from build123d import *

# Parameters (mm, degrees)
SKETCH1_R                 = 1.27
SKETCH1_R_2               = 1.5875
BOSS_EXTRUDE1_DEPTH       = 1.5875
CUT_EXTRUDE3_DEPTH        = 163.771012948
CUT_EXTRUDE4_DEPTH        = 163.771012948
F_8_0MM_DOWEL_HOLE1_D     = 8
F_8_0MM_DOWEL_HOLE1_DEPTH = 5.08
F_8_0MM_DOWEL_HOLE1_TIP   = 2.403442476


with BuildPart() as part:
    # Sketch1 → Boss-Extrude1 (new body)
    with BuildSketch(Plane(origin=(0, 0, 0), x_dir=(1, 0, 0), z_dir=(0, 1, 0))):
        with BuildLine():
            Line((-152.4, 43.5), (-152.4, -7.3))
            ThreePointArc((-152.4, -7.3), (-148.680256121, -16.280256121), (-139.7, -20))
            Line((-139.7, -20), (-61.723030548, -20))
            ThreePointArc((-61.723030548, -20), (-55.173880707, -21.818886254), (-50.500661357, -26.754545455))
            ThreePointArc((-50.500661357, -26.754545455), (57.15, 0), (-50.500661357, 26.754545455))
            ThreePointArc((-50.500661357, 26.754545455), (-55.173880707, 21.818886254), (-61.723030548, 20))
            Line((-61.723030548, 20), (-88.9, 20))
            ThreePointArc((-88.9, 20), (-97.880256121, 23.719743879), (-101.6, 32.7))
            Line((-101.6, 32.7), (-101.6, 43.5))
            ThreePointArc((-101.6, 43.5), (-105.319743879, 52.480256121), (-114.3, 56.2))
            Line((-114.3, 56.2), (-139.7, 56.2))
            ThreePointArc((-139.7, 56.2), (-148.680256121, 52.480256121), (-152.4, 43.5))
        make_face()
        with Locations(Location((-136.8, 0, 0), (0, 0, 270))):
            Circle(SKETCH1_R, mode=Mode.SUBTRACT)
        with Locations(Location((-117.2, 0, 0), (0, 0, 270))):
            Circle(SKETCH1_R, mode=Mode.SUBTRACT)
        with Locations(Location((0, 0, 0), (0, 0, 270))):
            Circle(SKETCH1_R_2, mode=Mode.SUBTRACT)
        with BuildLine():
            Line((-139.7, 33.02), (-114.3, 33.02))
            ThreePointArc((-114.3, 33.02), (-109.22, 38.1), (-114.3, 43.18))
            Line((-114.3, 43.18), (-139.7, 43.18))
            ThreePointArc((-139.7, 43.18), (-144.78, 38.1), (-139.7, 33.02))
        make_face(mode=Mode.SUBTRACT)
    extrude(amount=BOSS_EXTRUDE1_DEPTH)

    # Sketch5 → Cut-Extrude3 (cut, through all)
    with BuildSketch(Plane.XZ):
        with BuildLine():
            ThreePointArc((-19.811942673, -0.047660352), (-9.947246413, 17.133815477), (9.864696261, 17.18147583))
            ThreePointArc((9.864696261, 17.18147583), (14.025645813, 18.307134225), (12.899987418, 22.468083777))
            ThreePointArc((12.899987418, 22.468083777), (-13.007937617, 22.405758701), (-25.907925034, -0.062325076))
            ThreePointArc((-25.907925034, -0.062325076), (-22.852601492, -3.102983895), (-19.811942673, -0.047660352))
        make_face()
    extrude(amount=-CUT_EXTRUDE3_DEPTH, mode=Mode.SUBTRACT)

    # Sketch6 → Cut-Extrude4 (cut, through all)
    with BuildSketch(Plane.XZ):
        with BuildLine():
            Line((-16.102923339, -12.651081374), (-25.638527302, -29.167231918))
            ThreePointArc((-25.638527302, -29.167231918), (-26.310404552, -33.838744139), (-23.573299486, -37.683572006))
            Line((-23.573299486, -37.683572006), (-20.6375, -35.745198541))
            Line((-20.6375, -35.745198541), (-20.848318298, -39.257484944))
            ThreePointArc((-20.848318298, -39.257484944), (-17.010278569, -41.06644522), (-13.017246571, -42.501221061))
            Line((-13.017246571, -42.501221061), (-10.682756087, -39.86858848))
            Line((-10.682756087, -39.86858848), (-9.977344313, -43.315760417))
            ThreePointArc((-9.977344313, -43.315760417), (-5.801889244, -44.069724088), (-1.5735692, -44.422138399))
            Line((-1.5735692, -44.422138399), (0, -41.275))
            Line((0, -41.275), (1.5735692, -44.422138399))
            ThreePointArc((1.5735692, -44.422138399), (5.801889244, -44.069724088), (9.977344313, -43.315760417))
            Line((9.977344313, -43.315760417), (10.682756087, -39.86858848))
            Line((10.682756087, -39.86858848), (13.017246571, -42.501221061))
            ThreePointArc((13.017246571, -42.501221061), (17.010278569, -41.06644522), (20.848318298, -39.257484944))
            Line((20.848318298, -39.257484944), (20.6375, -35.745198541))
            Line((20.6375, -35.745198541), (23.573820101, -37.683915744))
            ThreePointArc((23.573820101, -37.683915744), (27.059445519, -35.264555976), (30.298513845, -32.523876749))
            Line((30.298513845, -32.523876749), (29.185832393, -29.185832393))
            Line((29.185832393, -29.185832393), (32.523876749, -30.298513845))
            ThreePointArc((32.523876749, -30.298513845), (35.264555976, -27.059445519), (37.683915744, -23.573820101))
            Line((37.683915744, -23.573820101), (35.745198541, -20.6375))
            Line((35.745198541, -20.6375), (39.257484944, -20.848318298))
            ThreePointArc((39.257484944, -20.848318298), (41.06644522, -17.010278569), (42.501221061, -13.017246571))
            Line((42.501221061, -13.017246571), (39.86858848, -10.682756087))
            Line((39.86858848, -10.682756087), (43.315760417, -9.977344313))
            ThreePointArc((43.315760417, -9.977344313), (44.069724088, -5.801889244), (44.422138399, -1.5735692))
            Line((44.422138399, -1.5735692), (41.275, 0))
            Line((41.275, 0), (44.421580406, 1.573290203))
            ThreePointArc((44.421580406, 1.573290203), (42.460414333, 5.866106656), (38.07882745, 7.62))
            Line((38.07882745, 7.62), (19.007619525, 7.62))
            ThreePointArc((19.007619525, 7.62), (14.370235205, 5.607875824), (12.67174635, 0.846666667))
            ThreePointArc((12.67174635, 0.846666667), (6.35, -10.998522628), (-7.069108017, -10.550720916))
            ThreePointArc((-7.069108017, -10.550720916), (-12.041680527, -9.641050833), (-16.102923339, -12.651081374))
        make_face()
    extrude(amount=-CUT_EXTRUDE4_DEPTH, mode=Mode.SUBTRACT)

    # Ø8.0mm Dowel Hole1
    with Locations(Plane(origin=(0, 1.5875, 0), x_dir=(1, 0, 0), z_dir=(0, 1, 0))):
        with Locations((-136.8, 0), (-117.2, 0)):
            Hole(F_8_0MM_DOWEL_HOLE1_D / 2, depth=F_8_0MM_DOWEL_HOLE1_DEPTH)
            with Locations((0, 0, -(F_8_0MM_DOWEL_HOLE1_DEPTH + F_8_0MM_DOWEL_HOLE1_TIP / 2))):  # 118° drill point
                Cone(0, F_8_0MM_DOWEL_HOLE1_D / 2, F_8_0MM_DOWEL_HOLE1_TIP, mode=Mode.SUBTRACT)


solid = part.part
Here's how the part is built. I have some questions about the finished solid (model axes, mm). A direction names the side the tool comes from. Round coordinates to 2 decimals unless told otherwise and drop trailing zeros. Loops run counter-clockwise (first coordinate to the right, second up) from the corner with the lowest first, then second, coordinate; pieces in that order, holes last.
1. If we section it at B-B on z = 14.5: Write out the boundary of the cut face in (x, y), plus the area to 3 significant figures.
Answer list:
outline: (-150.16, 0) - (-21.47, 0) - (-21.47, 1.59) - (-150.16, 1.59) - close; (-13.5, 0) - (55.28, 0) - (55.28, 1.59) - (-13.5, 1.59) - close
area: 313 mm2
2. Which directions (+Z, -Z, +X, -X, +Y, -Y) give clear straight access to the entire face, cutting with the end or side of a thin tool? Please do faces 1 (the face through (-49, 1.588, -1)), 2 (the face through (42.51, 0.78, 5.82)), 3 (the face through (-97.78, 0.78, -23.62)).
Answer list:
face 1: +Z, -Z, +X, -X, +Y
face 2: +Y, -Y
face 3: -Z, +Y, -Y
3. If we section it at A-A on x = -136.8: Write out the boundary of the cut face in (y, z).
Answer list:
outline: (0, -56.2) - (1.59, -56.2) - (1.59, -43.18) - (0, -43.18) - close; (0, -33.02) - (1.59, -33.02) - (1.59, -4) - (0, -4) - close; (0, 4) - (1.59, 4) - (1.59, 20) - (0, 20) - close
4. If we section it at C-C on x = -68: Write out the boundary of the cut face in (y, z).
Answer list:
outline: (0, -20) - (1.59, -20) - (1.59, 20) - (0, 20) - close
5. We'd pull the mould along X, two halves only. Please class faces 4 (the face through (-49, 0, -1)), 5 (the face through (-10.197, 0.783, 16.986)): +X half, -X half, draft (parallel to the pull), parting line (faces both ways), or undercut.
Answer list:
face 4: draft
face 5: undercut
6. If we section it at D-D on y = 0.55: Count the separate pieces of the cut face and the enclosed holes in it, plus the area to 3 significant figures.
Answer list:
separate pieces: 1
enclosed holes: 6
area: 12,800 mm2
7. If I drill on line 1 along Z through (x, y) = (-117.2, 0.8); line 2 along Z through (x, y) = (-139.5, 1); line 3 along X through (y, z) = (1.2, -23.5) (3 decimals), over which ranges is the centre line in solid material (lowest first)?
Answer list:
line 1: z = -56.2 to -43.18, -33.02 to -4, 4 to 20
line 2: z = -56.2 to -43.18, -33.02 to -2.95, 2.95 to 20
line 3: x = -152.4 to -97.655, -52.968 to -22.367, 37.635 to 52.095
8. For P1, Ø0.8, axis at x = -131, y = 1, coming from the -Z side; P2, Ø0.8, axis at y = 0.5, z = -40, coming from the +X side; P3, Ø0.5, axis at x = 25, y = 1, coming from the -Z side, each with a flat end and sliding along its axis, tell me the tip position at first contact or that it passes through.
Answer list:
P1: stops at z = -56.2
P2: stops at x = 41.21
P3: stops at z = -51.51
